from build123d import *

# Parameters (mm, degrees)
F1_DEPTH  = 30
F2_R      = 4.99999
F3_W      = 15
F3_H      = 15
F4_DEPTH  = 10
F5_W      = 15
F5_H      = 15
F6_DEPTH  = 10
F8_DEPTH  = 30
F10_DEPTH = 17.5
F12_DEPTH = 12.5
F14_DEPTH = 30


# Not quite as in the source:
# - a fillet or chamfer is up to 0.001 mm smaller than in the source, because OpenCascade refuses the exact size


with BuildPart() as f1:
    # F0 (on Front) → F1 (new body)
    with BuildSketch(Plane.XZ):
        Polygon((-25, -42.9761418055), (-25, -77.9761418055), (5, -77.9761418055), (5, 122.0238581945), (10, 122.0238581945), (10, 137.0238581945), (-30, 137.0238581945), (-30, 122.0238581945), (-25, 122.0238581945), (-25, 102.0238581945), (-20, 102.0238581945), (-20, 92.0238581945), (-25, 92.0238581945), (-25, 87.0238581945), (-20, 87.0238581945), (-20, 77.0238581945), (-25, 77.0238581945), (-25, 72.0238581945), (-20, 72.0238581945), (-20, 62.0238581945), (-25, 62.0238581945), (-25, 57.0238581945), (-20, 57.0238581945), (-20, 47.0238581945), (-25, 47.0238581945), (-25, 42.0238581945), (-20, 42.0238581945), (-20, 32.0238581945), (-25, 32.0238581945), (-25, 27.0238581945), (-20, 27.0238581945), (-20, 17.0238581945), (-25, 17.0238581945), (-25, 12.0238581945), (-20, 12.0238581945), (-20, 2.0238581945), (-25, 2.0238581945), (-25, -2.9761418055), (-20, -2.9761418055), (-20, -12.9761418055), (-25, -12.9761418055), (-25, -17.9761418055), (-20, -17.9761418055), (-20, -27.9761418055), (-25, -27.9761418055), (-25, -32.9761418055), (-20, -32.9761418055), (-20, -42.9761418055), align=None)
    extrude(amount=F1_DEPTH)

    # F2 (radius 5 in the source; OpenCascade refuses exactly that, so slightly less here)
    f2_edges = [f1.edges().sort_by_distance(p)[0] for p in [
        (-20, -15, 92.023858),
        (-20, -15, 77.023858),
        (-20, -15, 62.023858),
        (-20, -15, 47.023858),
        (-20, -15, 32.023858),
        (-20, -15, 17.023858),
        (-20, -15, 2.023858),
        (-20, -15, -12.976142),
        (-20, -15, -27.976142),
        (-20, -15, -42.976142),
    ]]
    fillet(f2_edges, radius=F2_R)

    # F3 (on face) → F4 (cut)
    with BuildSketch(Plane.XZ.offset(30)):
        Polygon((-15, -42.9761418055), (-20, -42.9761418055), (-20, -77.9761418055), (-5, -77.9761418055), (-5, 97.0238581945), (-15, 97.0238581945), align=None)
        with Locations((-12.5, 114.5238581945)):
            Rectangle(F3_W, F3_H)
    extrude(amount=-F4_DEPTH, mode=Mode.SUBTRACT)

    # F5 (on face) → F6 (cut)
    with BuildSketch(Plane(origin=(0, 0, 0), x_dir=(-1, 0, 0), z_dir=(0, 1, 0))):
        Polygon((20, -77.9761418055), (20, -42.9761418055), (15, -42.9761418055), (15, 96.101924777), (5, 96.101924777), (5, -77.9761418055), align=None)
        with Locations((12.5, 114.5238581945)):
            Rectangle(F5_W, F5_H)
    extrude(amount=-F6_DEPTH, mode=Mode.SUBTRACT)

    # F7 (on face) → F8 (join)
    with BuildSketch(Plane(origin=(0, 0, 0), x_dir=(-1, 0, 0), z_dir=(0, 1, 0))):
        Polygon((-30, 147.0238581945), (-30, 137.0238581945), (49.8739863932, 137.0238581945), (49.8739863932, 147.0238581945), (44.8739863932, 147.0238581945), (44.8739863932, 142.0238581945), (-25, 142.0238581945), (-25, 147.0238581945), align=None)
    extrude(amount=-F8_DEPTH)

    # F9 (on face) → F10 (join)
    with BuildSketch(Plane.XZ.offset(30)):
        with BuildLine():
            Line((-30, 137.0238581945), (-49.8739863932, 137.0238581945))
            ThreePointArc((-49.8739863932, 137.0238581945), (-42.4496519545, 126.1947551301), (-30, 122.0238581945))
            Line((-30, 122.0238581945), (-30, 137.0238581945))
        make_face()
        with BuildLine():
            ThreePointArc((10, 122.0238581945), (22.5, 126.1905248612), (30, 137.0238581945))
            Line((30, 137.0238581945), (10, 137.0238581945))
            Line((10, 137.0238581945), (10, 122.0238581945))
        make_face()
    extrude(amount=-F10_DEPTH)

    # F11 (on face) → F12 (cut)
    with BuildSketch(Plane.XZ.offset(30)):
        with BuildLine():
            Line((-30, 137.0238581945), (-49.8739863932, 137.0238581945))
            ThreePointArc((-49.8739863932, 137.0238581945), (-42.4496519545, 126.1947551301), (-30, 122.0238581945))
            Line((-30, 122.0238581945), (-30, 137.0238581945))
        make_face()
        with BuildLine():
            Line((10, 137.0238581945), (10, 122.0238581945))
            ThreePointArc((10, 122.0238581945), (22.5, 126.1905248612), (30, 137.0238581945))
            Line((30, 137.0238581945), (10, 137.0238581945))
        make_face()
    extrude(amount=-F12_DEPTH, mode=Mode.SUBTRACT)

    # F13 (on face) → F14 (cut)
    with BuildSketch(Plane(origin=(0, 0, 0), x_dir=(-1, 0, 0), z_dir=(0, 1, 0))):
        with BuildLine():
            Line((24.9369931966, 142.0238581945), (9.9369931966, 142.0238581945))
            Line((9.9369931966, 142.0238581945), (-5.0630068034, 142.0238581945))
            ThreePointArc((-5.0630068034, 142.0238581945), (9.9369931966, 139.7208182654), (24.9369931966, 142.0238581945))
        make_face()
    extrude(amount=-F14_DEPTH, mode=Mode.SUBTRACT)


solid = f1.part
For this review, take the finished solid that the model builds, in its own axes (mm). A direction names the side the tool comes from. Give positions to 0.01 mm unless a question says otherwise; leave off trailing zeros. Loops run counter-clockwise (first coordinate to the right, second up) from the corner with the lowest first, then second, coordinate; pieces in that order, holes last. Notation, with made-up numbers: (-2.5, 81.5) - (29.5, 81.5) arc R19 ccw to (29.5, 93.5) - close; hole circle Ø3 at (9, -14). An arc over 180 degrees is marked (long way). Write each question's results on one line, items separated by ' | '.
(1) For pin 1 Ø6 at (y, z) = (-19, 85.5) entering from -X; pin 2 Ø8 at (y, z) = (-22, 13.5) entering from +X; pin 3 Ø4 at (x, y) = (-6, -10) entering from +Z, all flat-tipped, find the tip position at first contact; note any pin that passes through.
Conclusion:
pin 1: x = -25 | pin 2: x = 5 | pin 3: z = 140.07
(2) Take a section at A-A (z = 120). Give the boundary of the cut face in (x, y), then the cut area to 3 significant figures.
Conclusion:
outline: (-25, -30) - (-20, -30) - (-20, -20) - (-5, -20) - (-5, -30) - (5, -30) - (5, 0) - (-5, 0) - (-5, -10) - (-20, -10) - (-20, 0) - (-25, 0) - close | area: 600 mm^2
(3) Draft analysis for pull direction X (two halves, no side actions). For faces 5 (the flat face through (25, -15, 144)), 6 (the flat face through (30, -15, 142)), 7 (the flat face through (20, -6, 137.024)), state which applies: +X half, -X half, draft (parallel to the pull), parting line (faces both ways), or undercut.
Conclusion:
face 5: undercut | face 6: +X half | face 7: draft
(4) Take a section at D-D (z = 29). Give the boundary of the cut face in (x, y), then the cut area to 3 significant figures.
Conclusion:
outline: (-25, -30) - (-15, -30) - (-15, -20) - (-5, -20) - (-5, -30) - (5, -30) - (5, 0) - (-5, 0) - (-5, -10) - (-15, -10) - (-15, 0) - (-25, 0) - close | area: 700 mm^2
(5) For line 1 along X through (y, z) = (-4.5, -59); line 2 along Z through (x, y) = (19, -7); line 3 along X through (y, z) = (-24.5, 93.5), list the stretches that pass through material, from the lowest coordinate up.
Conclusion:
line 1: -25 to -20, -5 to 5 | line 2: 137.02 to 142.02 | line 3: -21.45 to -15, -5 to 5
(6) For faces 1 (the flat face through (-25, -15, -15)), 2 (the flat face through (-20, -25, 114)), 3 (the flat face through (-15, -25, 28)), 4 (the flat face through (-23, -15, -17.976)), list the 3-axis set-ups (+Z, -Z, +X, -X, +Y, -Y) from which the entire face can be reached by the end or side of a thin tool; tool diameter is ignored.
Conclusion:
face 1: -Z, -X, +Y, -Y | face 2: -Y | face 3: -Z, -Y | face 4: -X, +Y, -Y
(7) Take a section at C-C (x = -22). State how many separate pieces and enclosed holes the cut face has, then the cut area to 3 significant figures.
Conclusion:
separate pieces: 11 | enclosed holes: 0 | area: 3,880 mm^2
(8) Take a section at B-B (x = -37). Give the boundary of the cut face in (y, z), then the cut area to 3 significant figures.
Conclusion:
outline: (-30, 137.02) - (-17.5, 137.02) - (-17.5, 123.25) - (-12.5, 123.25) - (-12.5, 137.02) - (0, 137.02) - (0, 142.02) - (-30, 142.02) - close | area: 219 mm^2
